Can you work these out from the model? Positions are in its coordinate system, mm. A direction names the side the tool comes from. Give positions to 0.01 mm unless a question says otherwise; leave off trailing zeros. Loops run counter-clockwise (first coordinate to the right, second up) from the corner with the lowest first, then second, coordinate; pieces in that order, holes last.
from build123d import *

# Parameters (mm, degrees)
SKETCH1_W           = 40.05
SKETCH1_H           = 50
BOSS_EXTRUDE1_DEPTH = 4
SKETCH2_W           = 24
SKETCH2_H           = 58
BOSS_EXTRUDE2_DEPTH = 8
SKETCH4_W           = 24
SKETCH4_H           = 58
BOSS_EXTRUDE3_DEPTH = 8
BOSS_EXTRUDE5_DEPTH = 40.05
SKETCH6_W           = 32.05
SKETCH6_H           = 50
CUT_EXTRUDE1_DEPTH  = 8
SKETCH7_R           = 2
CUT_EXTRUDE2_DEPTH  = 8
SKETCH9_R           = 2
CUT_EXTRUDE3_DEPTH  = 50
SKETCH11_W          = 16
SKETCH11_H          = 50
CUT_EXTRUDE4_DEPTH  = 80


with BuildPart() as part:
    # Sketch1 → Boss-Extrude1 (new, symmetric)
    with BuildSketch(Plane.XY):
        Rectangle(SKETCH1_W, SKETCH1_H)
    extrude(amount=BOSS_EXTRUDE1_DEPTH, both=True)

    # Sketch2 → Boss-Extrude2 (add)
    with BuildSketch(Plane(origin=(20.025, 0, 0), x_dir=(0, 0, -1), z_dir=(1, 0, 0))):
        with Locations((8, 4)):
            Rectangle(SKETCH2_W, SKETCH2_H)
    extrude(amount=BOSS_EXTRUDE2_DEPTH)

    # Sketch4 → Boss-Extrude3 (add)
    with BuildSketch(Plane.ZY.offset(20.025)):
        with Locations((-8, 4)):
            Rectangle(SKETCH4_W, SKETCH4_H)
    extrude(amount=BOSS_EXTRUDE3_DEPTH)

    # Sketch5 → Boss-Extrude5 (add)
    with BuildSketch(Plane.ZY.offset(-20.025)):
        Polygon((-20, -25), (-20, 33), (4, 33), (4, 25), (-12.05, 25), (-12.05, -25), align=None)
    extrude(amount=BOSS_EXTRUDE5_DEPTH)

    # Sketch6 → Cut-Extrude1 (cut)
    with BuildSketch(Plane(origin=(0, 0, -20), x_dir=(-1, 0, 0), z_dir=(0, 0, -1))):
        Rectangle(SKETCH6_W, SKETCH6_H)
    extrude(amount=-CUT_EXTRUDE1_DEPTH, mode=Mode.SUBTRACT)

    # Sketch7 → Cut-Extrude2 (cut)
    with BuildSketch(Plane(origin=(0, 33, 0), x_dir=(1, 0, 0), z_dir=(0, 1, 0))):
        with Locations(Location((0, 8, 0), (0, 0, 270))):
            Circle(SKETCH7_R)
    extrude(amount=-CUT_EXTRUDE2_DEPTH, mode=Mode.SUBTRACT)

    # Sketch9 → Cut-Extrude3 (cut, symmetric)
    with BuildSketch(Plane.ZY.offset(-20.025)):
        with Locations((-8.025, 0)):
            Circle(SKETCH9_R)
    extrude(amount=CUT_EXTRUDE3_DEPTH, both=True, mode=Mode.SUBTRACT)

    # Sketch11 → Cut-Extrude4 (cut)
    with BuildSketch(Plane(origin=(28.025, 0, 0), x_dir=(0, 0, -1), z_dir=(1, 0, 0))):
        with Locations((12, 0)):
            Rectangle(SKETCH11_W, SKETCH11_H)
    extrude(amount=-CUT_EXTRUDE4_DEPTH, mode=Mode.SUBTRACT)


solid = part.part
(1) Suppose I cut it at D-D on z = -17.5. List the corners of the cut face in (x, y) for me (3 decimals).
Returned:
outline: (-28.025, 25) - (28.025, 25) - (28.025, 33) - (-28.025, 33) - close
(2) Suppose I cut it at A-A on z = -8. List the corners of the cut face in (x, y) for me (3 decimals), plus the area to 3 significant figures.
Returned:
outline: (-28.025, 25) - (-2, 25) - (-2, 33) - (-28.025, 33) - close; (2, 25) - (28.025, 25) - (28.025, 33) - (2, 33) - close
area: 416 mm2
(3) Please list where these lines run through material, in increasing order: probe 1 along X at (y, z) = (30.5, -8) (3 decimals); probe 2 along Z at (x, y) = (1.5, -2); probe 3 along Y at (x, z) = (-10, -14.75).
Returned:
probe 1: x = -28.025 to -2, 2 to 28.025
probe 2: z = -4 to 4
probe 3: y = 25 to 33
(4) Which directions (+Z, -Z, +X, -X, +Y, -Y) give clear straight access to the entire face, cutting with the end or side of a thin tool? Please do faces 1 (the flat face through (0, 0, -4)), 2 (the flat face through (0, 29, -20)).
Returned:
face 1: -Z, +X, -X, -Y
face 2: -Z, +X, -X, +Y, -Y
(5) Suppose I cut it at B-B on x = 0. List the corners of the cut face in (y, z) for me.
Returned:
outline: (-25, -4) - (25, -4) - (25, -6) - (33, -6) - (33, 4) - (-25, 4) - close; (25, -20) - (33, -20) - (33, -10) - (25, -10) - close
(6) Thinking about a two-plate mould opening in Z: for faces 3 (the cylindrical face through (-1.2, 29.1, -9.6)), 4 (the flat face through (0, 4, 4)), 5 (the flat face through (0, -25, 0)), which applies, pulls with the +Z half, pulls with the -Z half, needs draft (parallel to the pull), parting line crosses it, or undercut?
Returned:
face 3: undercut
face 4: pulls with the +Z half
face 5: needs draft
(7) Will these pins go through, and if not, where does the flat tip stop? P1, Ø4, axis at x = 11, z = -7, coming from the -Y side; P2, Ø5, axis at x = -6, y = 7, coming from the -Z side; P3, Ø8, axis at y = 19, z = -10.5, coming from the -X side.
Returned:
P1: stops at y = 25
P2: stops at z = -4
P3: passes through
(8) Suppose I cut it at C-C on y = 11. List the corners of the cut face in (x, z) for me (3 decimals), plus the area to 3 significant figures.
Returned:
outline: (-28.025, -4) - (28.025, -4) - (28.025, 4) - (-28.025, 4) - close
area: 448 mm2
